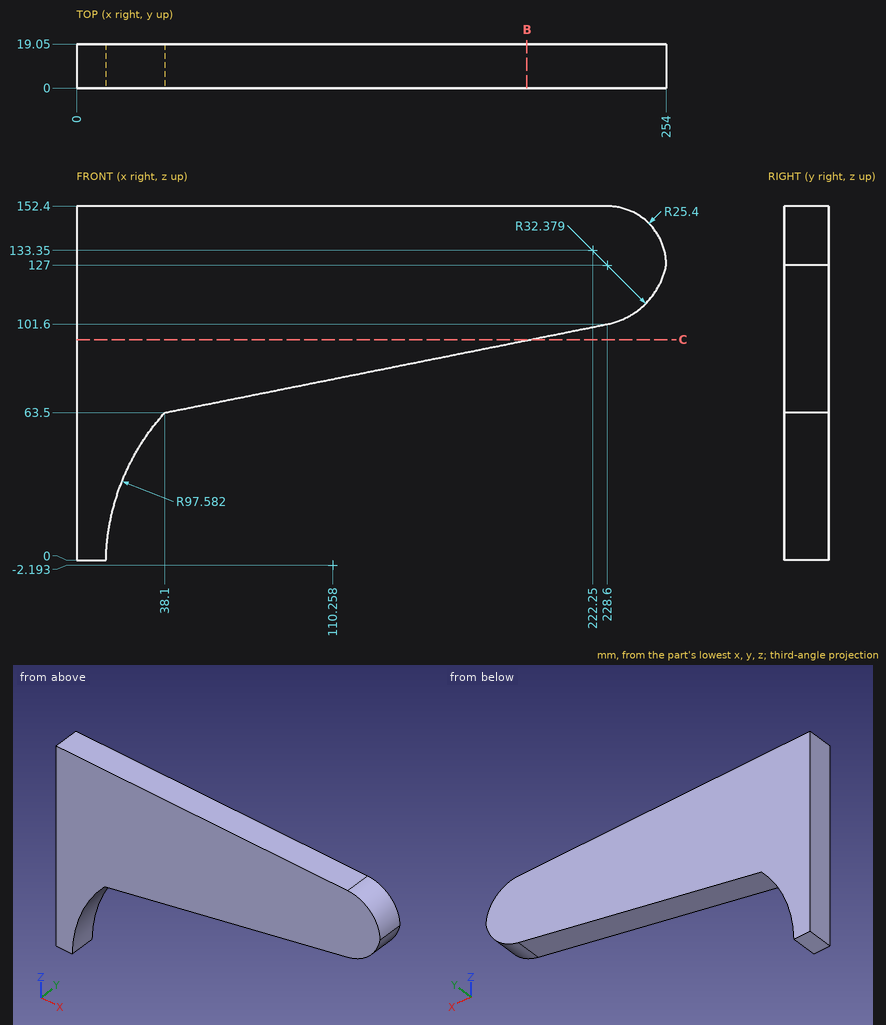
Print and shaded views of the part. All mm, measured from the part's lowest x, y and z. Give positions to 0.01 mm unless a question says otherwise; leave off trailing zeros. Loops run counter-clockwise (first coordinate to the right, second up) from the corner with the lowest first, then second, coordinate; pieces in that order, holes last. Notation, with made-up numbers: (80.25, 63) -> (106.25, 63) arc R17 ccw to (106.25, 76) -> close; hole circle Ø8 at (4.25, 40). An arc over 180 degrees is marked (long way). Answer in a Markdown table with one row per item.
Item 1: Flat gauge pins, fed straight in: P1, Ø8, axis at x = 29.5, z = 47, coming from the -Y side; P2, Ø3, axis at x = 201.5, y = 16, coming from the -Z side; P3, Ø1.5, axis at y = 8.5, z = 32.5, coming from the +X side; P4, Ø8, axis at y = 13, z = 23.5, coming from the +X side. Where does each tip first touch, or does it go through?
Findings below:
| item | result |
|---|---|
| P1 | stops at y = 0 |
| P2 | stops at z = 95.88 |
| P3 | stops at x = 19.34 |
| P4 | stops at x = 17.3 |
Item 2: Slice it at C-C on z = 95. Write the cut outline in (x, y).
Findings below:
| item | result |
|---|---|
| outline | (0, 0) -> (195.6, 0) -> (195.6, 19.05) -> (0, 19.05) -> close |
Item 3: Probe line 1 along X through (y, z) = (1, 135.5) (1 decimal); line 2 along X through (y, z) = (4.5, 49); line 3 along Z through (x, y) = (146.5, 9.75). List the from-to ranges inside material, lowest first. Write a range as [from, to].
Findings below:
| item | result |
|---|---|
| line 1 | x = [0, 252.5] |
| line 2 | x = [0, 27.18] |
| line 3 | z = [85.18, 152.4] |
Item 4: Slice it at B-B on x = 194. Write the cut outline in (y, z).
Findings below:
| item | result |
|---|---|
| outline | (0, 94.68) -> (19.05, 94.68) -> (19.05, 152.4) -> (0, 152.4) -> close |
